from build123d import *

# Parameters (mm, degrees)
F1_ANGLE = 335
F2_R     = 2.082692


with BuildPart() as f1:
    # F0 (on Right) → F1 (revolve)
    with BuildSketch(Plane.YZ):
        with BuildLine():
            Line((17.637674, 43.847844), (0, 43.847844))
            Line((0, 43.847844), (0, 0))
            Line((0, 0), (17.637674, 0))
            ThreePointArc((17.637674, 0), (16.761053, 11.513244), (12.316811, 22.170259))
            ThreePointArc((12.316811, 22.170259), (12.001861, 33.739372), (17.637674, 43.847844))
        make_face()
    revolve(axis=Axis((0, 0, 21.923922), (0, 0, -1)), revolution_arc=F1_ANGLE)

    # F2
    f2_edges = [f1.edges().sort_by_distance(p)[0] for p in [
        (3.817491, -17.21959, 43.847844),
        (3.817491, -17.21959, 0),
    ]]
    fillet(f2_edges, radius=F2_R)


solid = f1.part
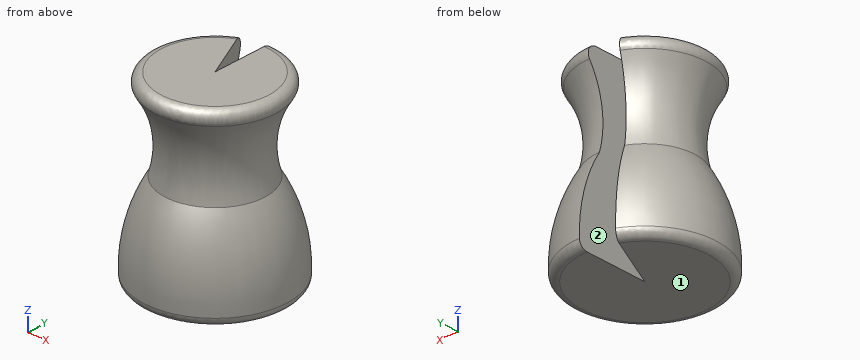
For this review, take the finished solid that the model builds, in its own axes (mm). Face numbers are marked on the shaded views. Give positions to 0.01 mm unless a question says otherwise; leave off trailing zeros. Loops run counter-clockwise (first coordinate to the right, second up) from the corner with the lowest first, then second, coordinate; pieces in that order, holes last.
Item 1: Take a section at A-A, the plane z = 36. State the section outline as (x, y) points, and give its area (3 significant figures).
Item 2: For line 1 along Y through (x, z) = (2.5, 15.5); line 2 along X through (y, z) = (1.5, 18.5); line 3 along X through (y, z) = (6.5, 18), list the stretches that pass through material, from the lowest coordinate up.
Item 3: Take a section at B-B, the plane z = 28. State the section outline as (x, y) points.
Item 4: Insertion check: pin 1 (8 mm diameter, centred on x = 13.5, z = 17.5, fed in from -Y); pin 2 (5 mm diameter, centred on x = -8.5, z = 34, fed in from +Y); pin 3 (10 mm diameter, centred on y = 6.5, z = 6, fed in from -X). Each pin has a flat end and moves straight along its axis. Give the tip position at first contact, or say it passes through.
Item 5: Draft analysis for pull direction X (two halves, no side actions). For the marked faces 1 and 2, state which applies: +X half, -X half, draft (parallel to the pull), parting line (faces both ways), or undercut.
Calculated:
1. outline: (-5.36, 11.5) arc R12.69 ccw (long way) to (0, 12.69) - (0, 0) - close
1. area: 471 mm2
2. line 1: y = -15.36 to 15.36
2. line 2: x = -14.23 to -0.7, 0 to 14.23
2. line 3: x = -13.01 to -3.03, 0 to 13.01
3. outline: (-4.81, 10.31) arc R11.38 ccw (long way) to (0, 11.38) - (0, 0) - close
4. pin 1: stops at y = -11.89
4. pin 2: stops at y = 10.7
4. pin 3: stops at x = -17.65
5. face 1: draft
5. face 2: undercut
